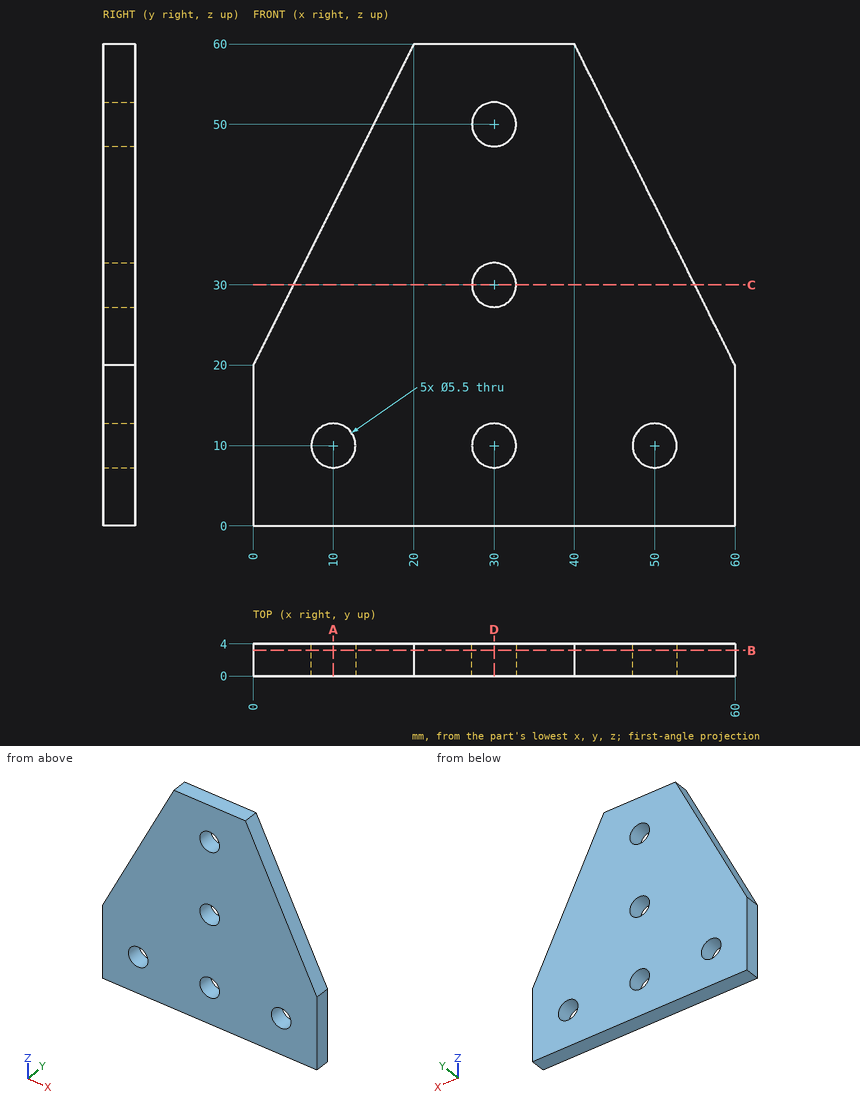
Geometry check sheet. Reference: drawing and pictorial views, mm from the part's lowest x, y, z. Round coordinates to 2 decimals unless told otherwise and drop trailing zeros. Loops run counter-clockwise (first coordinate to the right, second up) from the corner with the lowest first, then second, coordinate; pieces in that order, holes last. Notation, with made-up numbers: (39.25, -21) -> (58.25, -21) arc R22 cw to (58.25, 18) -> close; hole circle Ø3 at (9.5, 76). An arc over 180 degrees is marked (long way). Answer as a JSON object with one key per item and string values.
Q1. Scan lines: line 1 (Z direction, x = 30, y = 2.9); line 2 (Z direction, x = 28.5, y = 3.1); line 3 (Z direction, x = 10, y = 1.85). Record each from-to range of solid material in increasing order. Write a range as from..to.
Data:
{"line 1": "z = 0..7.25, 12.75..27.25, 32.75..47.25, 52.75..60", "line 2": "z = 0..7.7, 12.3..27.7, 32.3..47.7, 52.3..60", "line 3": "z = 0..7.25, 12.75..40"}
Q2. Section check C-C (z = 30). Record the boundary of the cut face in (x, y), then the cut area to 3 significant figures.
Data:
{"outline": "(5, 0) -> (27.25, 0) -> (27.25, 4) -> (5, 4) -> close; (32.75, 0) -> (55, 0) -> (55, 4) -> (32.75, 4) -> close", "area": "178 mm2"}
Q3. Section check D-D (x = 30). Record the boundary of the cut face in (y, z), then the cut area to 3 significant figures.
Data:
{"outline": "(0, 0) -> (4, 0) -> (4, 7.25) -> (0, 7.25) -> close; (0, 12.75) -> (4, 12.75) -> (4, 27.25) -> (0, 27.25) -> close; (0, 32.75) -> (4, 32.75) -> (4, 47.25) -> (0, 47.25) -> close; (0, 52.75) -> (4, 52.75) -> (4, 60) -> (0, 60) -> close", "area": "174 mm2"}
Q4. Section check A-A (x = 10). Record the boundary of the cut face in (y, z), then the cut area to 3 significant figures.
Data:
{"outline": "(0, 0) -> (4, 0) -> (4, 7.25) -> (0, 7.25) -> close; (0, 12.75) -> (4, 12.75) -> (4, 40) -> (0, 40) -> close", "area": "138 mm2"}
Q5. Go/stop test with flat-tipped pins: P1, Ø4, axis at x = 25, z = 13, coming from the -Y side; P2, Ø1.5, axis at y = 2, z = 40, coming from the +X side (3 decimals); P3, Ø1, axis at x = 42, y = 2.5, coming from the +Z side. Record where each tip stops, or that it passes through.
Data:
{"P1": "stops at y = 0", "P2": "stops at x = 50.375", "P3": "stops at z = 57"}
Q6. Section check B-B (y = 3.2). Record the boundary of the cut face in (x, z).
Data:
{"outline": "(0, 0) -> (60, 0) -> (60, 20) -> (40, 60) -> (20, 60) -> (0, 20) -> close; hole circle Ø5.5 at (10, 10); hole circle Ø5.5 at (30, 10); hole circle Ø5.5 at (30, 30); hole circle Ø5.5 at (30, 50); hole circle Ø5.5 at (50, 10)"}
